Model file for the job. Use its own axes, mm. A direction names the side the tool comes from. Round coordinates to 2 decimals unless told otherwise and drop trailing zeros. Order: outer loops, then holes, each group sorted by start corner. A loop starts at its lowest first (then second) coordinate and runs counter-clockwise, first axis right, second up. Notation, with made-up numbers: (-4, -11.75) -> (53, -11.75) arc R14 cw to (53, 14.25) -> close; hole circle Ø9 at (60.25, 71). An arc over 180 degrees is marked (long way). Put each result on its own line as item: value. Start each with the question number.
Q1. Cut at D-D, the plane y = -8.89. List the corners of the cut face in (x, z).
Q2. Pull direction X, two halves, no side cores. Call faces 1 (the face through (10.902, 3.433, 26.332)), 2 (the face through (10, -10, 2.54)), 3 (the face through (17.744, -9.863, 1.252)): released by +X, released by -X, zero draft, split by the parting line, or undercut.
Q3. Flat gauge pins, fed straight in: P1, Ø3, axis at x = -5.5, y = 14.5, coming from the +Z side; P2, Ø5, axis at x = -11, z = 22, coming from the -Y side; P3, Ø10, axis at y = -11.5, z = 20.5, coming from the +X side; P4, Ø3, axis at x = 15.4, y = -8.89, coming from the +Z side. Where does each tip first touch, or does it go through?
Q4. Probe L1, parallel to X at y = -8, z = 1; L2, parallel to Y at x = 0, z = 40.5; L3, parallel to Z at x = 20.5, y = 7. List the from-to ranges inside material, lowest first.
Q5. Cut at A-A, the plane y = 0. List the corners of the cut face in (x, z) (3 decimals).
Q6. Cut at C-C, the plane y = 17.78. List the corners of the cut face in (x, z) (3 decimals).
Q7. 3-axis set-ups, long thin cutter, end or side, ignore diameter. For faces 4 (the face through (-0.55, 15.3, 1.25)), 5 (the face through (-9.273, 6.057, 20.957)): which of +Z, -Z, +X, -X, +Y, -Y reach the whole face in a straight line?
Q8. Cut at B-B, the plane x = 0. List the corners of the cut face in (y, z) (3 decimals).
from build123d import *

# Parameters (mm, degrees)
F0_R     = 11.43
F0_R_2   = 10.16
F1_DEPTH = 50.8
F0_R_3   = 22.225
F0_R_4   = 2.54
F2_DEPTH = 2.54
F3_R     = 6.35
F4_DEPTH = 12.7


with BuildPart() as f1:
    # F0 (on Top) → F1 (new body)
    with BuildSketch(Plane.XY):
        Circle(F0_R)
        Circle(F0_R_2, mode=Mode.SUBTRACT)
    extrude(amount=F1_DEPTH)

    # F0 (on Top) → F2 (join)
    with BuildSketch(Plane.XY):
        Circle(F0_R_3)
        with Locations((-15.397932, -8.89)):
            Circle(F0_R_4, mode=Mode.SUBTRACT)
        with Locations((15.397932, -8.89)):
            Circle(F0_R_4, mode=Mode.SUBTRACT)
        Circle(F0_R, mode=Mode.SUBTRACT)
        with Locations((0, 17.78)):
            Circle(F0_R_4, mode=Mode.SUBTRACT)
    extrude(amount=F2_DEPTH)

    # F3 (on Right) → F4 (cut)
    with BuildSketch(Plane.YZ):
        with Locations((0, 19.05)):
            Circle(F3_R)
    extrude(amount=-F4_DEPTH, mode=Mode.SUBTRACT)


solid = f1.part
Ans:
1. outline: (-20.37, 0) -> (-17.94, 0) -> (-17.94, 2.54) -> (-20.37, 2.54) -> close; (-12.86, 0) -> (-4.92, 0) -> (-4.92, 50.8) -> (-7.18, 50.8) -> (-7.18, 2.54) -> (-12.86, 2.54) -> close; (4.92, 0) -> (12.86, 0) -> (12.86, 2.54) -> (7.18, 2.54) -> (7.18, 50.8) -> (4.92, 50.8) -> close; (17.94, 0) -> (20.37, 0) -> (20.37, 2.54) -> (17.94, 2.54) -> close
2. face 1: split by the parting line
2. face 2: zero draft
2. face 3: undercut
3. P1: stops at z = 2.54
3. P2: stops at y = -7.64
3. P3: stops at x = 9.4
3. P4: passes through
4. L1: x = -20.74 to -17.78, -13.02 to -6.26, 6.26 to 13.02, 17.78 to 20.74
4. L2: y = -11.43 to -10.16, 10.16 to 11.43
4. L3: z = 0 to 2.54
5. outline: (-22.225, 0) -> (-10.16, 0) -> (-10.16, 12.7) -> (-11.43, 12.7) -> (-11.43, 2.54) -> (-22.225, 2.54) -> close; (-11.43, 25.4) -> (-10.16, 25.4) -> (-10.16, 50.8) -> (-11.43, 50.8) -> close; (10.16, 0) -> (22.225, 0) -> (22.225, 2.54) -> (11.43, 2.54) -> (11.43, 50.8) -> (10.16, 50.8) -> close
6. outline: (-13.335, 0) -> (-2.54, 0) -> (-2.54, 2.54) -> (-13.335, 2.54) -> close; (2.54, 0) -> (13.335, 0) -> (13.335, 2.54) -> (2.54, 2.54) -> close
7. face 4: +Z, -Z
7. face 5: -X
8. outline: (-22.225, 0) -> (-10.16, 0) -> (-10.16, 50.8) -> (-11.43, 50.8) -> (-11.43, 2.54) -> (-22.225, 2.54) -> close; (10.16, 0) -> (15.24, 0) -> (15.24, 2.54) -> (11.43, 2.54) -> (11.43, 50.8) -> (10.16, 50.8) -> close; (20.32, 0) -> (22.225, 0) -> (22.225, 2.54) -> (20.32, 2.54) -> close
